from build123d import *

# Parameters (mm, degrees)
SKETCH1_W           = 30
SKETCH1_H           = 30
BOSS_EXTRUDE1_DEPTH = 4
SKETCH2_R           = 5
SKETCH2_W           = 10
SKETCH2_H           = 10
CUT_EXTRUDE1_DEPTH  = 5
FILLET1_R           = 5
CUT_EXTRUDE2_DEPTH  = 20
CUT_EXTRUDE3_DEPTH  = 20


with BuildPart() as part:
    # Sketch1 → Boss-Extrude1 (new body)
    with BuildSketch(Plane(origin=(0, 0, 0), x_dir=(1, 0, 0), z_dir=(0, 1, 0))):
        with Locations((15, 15)):
            Rectangle(SKETCH1_W, SKETCH1_H)
    extrude(amount=BOSS_EXTRUDE1_DEPTH)

    # Sketch2 → Cut-Extrude1 (cut, through all)
    with BuildSketch(Plane(origin=(0, 4, 0), x_dir=(1, 0, 0), z_dir=(0, 1, 0))):
        with Locations(Location((8, 10, 0), (0, 0, 270))):  # turned: the seam where the file's is
            Circle(SKETCH2_R)
        with Locations((18, 22)):
            Rectangle(SKETCH2_W, SKETCH2_H)
    extrude(amount=-CUT_EXTRUDE1_DEPTH, mode=Mode.SUBTRACT)

    # Fillet1
    fillet1_edges = [part.edges().sort_by_distance(p)[0] for p in [
        (0, 2, -30),
    ]]
    fillet(fillet1_edges, radius=FILLET1_R)

    # Sketch3 → Cut-Extrude2 (cut)
    with BuildSketch(Plane(origin=(30, 0, 0), x_dir=(0, 0, -1), z_dir=(1, 0, 0))):
        Polygon((0, 0), (4, 4), (0, 4), align=None)
    extrude(amount=-CUT_EXTRUDE2_DEPTH, mode=Mode.SUBTRACT)

    # Sketch4 → Cut-Extrude3 (cut)
    with BuildSketch(Plane.XY):
        Polygon((30, 4), (26, 0), (30, 0), align=None)
    extrude(amount=-CUT_EXTRUDE3_DEPTH, mode=Mode.SUBTRACT)


solid = part.part
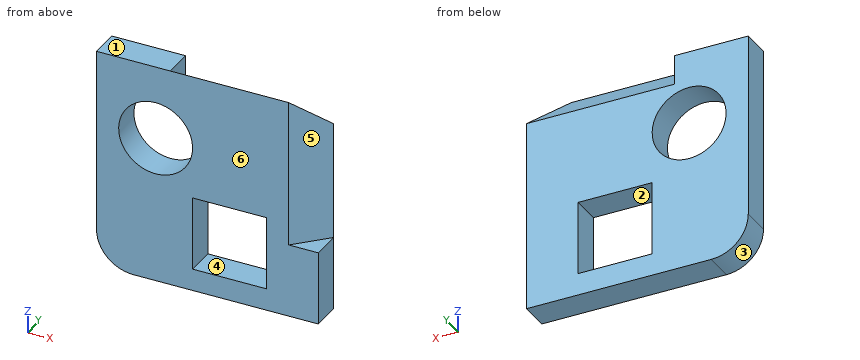
CAD build for the part. Positions are in the model's coordinates, mm. Face numbers are marked on the shaded views. A direction names the side the tool comes from. Give positions to 0.01 mm unless a question says otherwise; leave off trailing zeros. Loops run counter-clockwise (first coordinate to the right, second up) from the corner with the lowest first, then second, coordinate; pieces in that order, holes last. Notation, with made-up numbers: M 63.5,-33.5 L 117.5,-33.5 A26 ccw 117.5,1.5 Z; hole C -6.75,18 d8. An arc over 180 degrees is marked long. One line per question, with ' | ' between items. Start each with the question number.
1. Two-plate mould, pull along Z, no slides. Class the marked faces 1, 2 and 3: pulls with the +Z half, pulls with the -Z half, needs draft (parallel to the pull), parting line crosses it, or undercut.
2. Saw through at A-A on z = -18.75. Give the cut face in (x, y).
3. Saw through at B-B on x = 19.75. Give the cut face in (y, z).
4. Flat gauge pins, fed straight in: pin 1 (5 mm diameter, centred on x = 13, z = -10.5, fed in from -Y); pin 2 (2 mm diameter, centred on x = 26, y = 3, fed in from +Z); pin 3 (9 mm diameter, centred on x = 8, z = -10, fed in from +Y). Where does each tip first touch, or does it go through?
5. Saw through at C-C on y = 2.6. Give the cut face in (x, z), plus the area to 3 significant figures.
6. 3-axis set-ups, long thin cutter, end or side, ignore diameter. For the marked faces 4, 5 and 6: which of +Z, -Z, +X, -X, +Y, -Y reach the whole face in a straight line?
7. Saw through at D-D on x = 24. Give the cut face in (y, z).
8. Probe L1, parallel to X at y = 2, z = -24.25; L2, parallel to Y at x = 17.75, z = -3; L3, parallel to X at y = 2.3, z = -10. List the from-to ranges inside material, lowest first. Write a range as from..to.
Result sheet:
1) face 1: pulls with the +Z half | face 2: undercut | face 3: pulls with the -Z half
2) outline: M 0,0 L 13,0 L 13,4 L 0,4 Z; M 23,0 L 26,0 L 30,4 L 23,4 Z
3) outline: M 0,-30 L 4,-30 L 4,-27 L 0,-27 Z; M 0,-17 L 4,-17 L 4,-4 L 0,0 Z
4) pin 1: stops at y = 0 | pin 2: stops at z = -2 | pin 3: passes through
5) outline: M 0,-25 A5 ccw 5,-30 L 30,-30 L 30,-20 L 28.6,-20 L 28.6,-2.6 L 10,-2.6 L 10,0 L 0,0 Z; hole C 8,-10 d10; hole M 13,-27 L 23,-27 L 23,-17 L 13,-17 Z | area: 640 mm^2
6) face 4: +Y, -Y | face 5: +Z, +X, -Y | face 6: +Z, -Z, +X, -X, -Y
7) outline: M 0,-30 L 4,-30 L 4,-4 L 0,0 Z
8) L1: x = 0..13, 23..30 | L2: y = 0..3 | L3: x = 0..3, 13..28.3
